from build123d import *

# Parameters (mm, degrees)
RESSALTO_EXTRUS_O1_DEPTH = 37.5


with BuildPart() as part:
    # Esboço1 → Ressalto-extrusão1 (new body, symmetric)
    with BuildSketch(Plane.XY):
        with BuildLine():
            Line((-6, -8.507783687), (-6, -6.707106781))
            Line((-6, -6.707106781), (-4.292893219, -5))
            Line((-4.292893219, -5), (-0.866025404, -5))
            Line((-0.866025404, -5), (0, -4.5))
            Line((0, -4.5), (0.866025404, -5))
            Line((0.866025404, -5), (4.292893219, -5))
            Line((4.292893219, -5), (6, -6.707106781))
            Line((6, -6.707106781), (6, -8.507783687))
            Line((6, -8.507783687), (2.3, -8.507783687))
            Line((2.3, -8.507783687), (2.3, -9.253891844))
            Line((2.3, -9.253891844), (3, -9.253891844))
            Line((3, -9.253891844), (3, -10))
            Line((3, -10), (8.85, -10))
            ThreePointArc((8.85, -10), (9.663172798, -9.663172798), (10, -8.85))
            Line((10, -8.85), (10, -3))
            Line((10, -3), (9.253891844, -3))
            Line((9.253891844, -3), (9.253891844, -2.3))
            Line((9.253891844, -2.3), (8.507783687, -2.3))
            Line((8.507783687, -2.3), (8.507783687, -6))
            Line((8.507783687, -6), (6.707106781, -6))
            Line((6.707106781, -6), (5, -4.292893219))
            Line((5, -4.292893219), (5, -0.867675042))
            Line((5, -0.867675042), (4.502666183, 0))
            Line((4.502666183, 0), (5, 0.866025404))
            Line((5, 0.866025404), (5, 4.292893219))
            Line((5, 4.292893219), (6.707106781, 6))
            Line((6.707106781, 6), (8.507783687, 6))
            Line((8.507783687, 6), (8.507783687, 3))
            Line((8.507783687, 3), (9.253891844, 3))
            Line((9.253891844, 3), (10, 3))
            Line((10, 3), (10, 8.85))
            ThreePointArc((10, 8.85), (9.663172798, 9.663172798), (8.85, 10))
            Line((8.85, 10), (3, 10))
            Line((3, 10), (3, 9.253891844))
            Line((3, 9.253891844), (2.3, 9.253891844))
            Line((2.3, 9.253891844), (2.3, 8.507783687))
            Line((2.3, 8.507783687), (6, 8.507783687))
            Line((6, 8.507783687), (6, 6.707106781))
            Line((6, 6.707106781), (4.292893219, 5))
            Line((4.292893219, 5), (0.866025404, 5))
            Line((0.866025404, 5), (0, 4.502147794))
            Line((0, 4.502147794), (-0.866025404, 5))
            Line((-0.866025404, 5), (-4.292893219, 5))
            Line((-4.292893219, 5), (-6, 6.707106781))
            Line((-6, 6.707106781), (-6, 8.507783687))
            Line((-6, 8.507783687), (-2.3, 8.507783687))
            Line((-2.3, 8.507783687), (-2.3, 9.253891844))
            Line((-2.3, 9.253891844), (-3, 9.253891844))
            Line((-3, 9.253891844), (-3, 10))
            Line((-3, 10), (-8.85, 10))
            ThreePointArc((-8.85, 10), (-9.663172798, 9.663172798), (-10, 8.85))
            Line((-10, 8.85), (-10, 3))
            Line((-10, 3), (-9.253891844, 3))
            Line((-9.253891844, 3), (-9.253891844, 2.3))
            Line((-9.253891844, 2.3), (-8.507783687, 2.3))
            Line((-8.507783687, 2.3), (-8.507783687, 6))
            Line((-8.507783687, 6), (-6.707106781, 6))
            Line((-6.707106781, 6), (-5, 4.292893219))
            Line((-5, 4.292893219), (-5, 0.866025404))
            Line((-5, 0.866025404), (-4.498098017, -0.000824819))
            Line((-4.498098017, -0.000824819), (-5, -0.867675042))
            Line((-5, -0.867675042), (-5, -4.292893219))
            Line((-5, -4.292893219), (-6.707106781, -6))
            Line((-6.707106781, -6), (-8.507783687, -6))
            Line((-8.507783687, -6), (-8.507783687, -2.3))
            Line((-8.507783687, -2.3), (-9.253891844, -2.3))
            Line((-9.253891844, -2.3), (-9.253891844, -3))
            Line((-9.253891844, -3), (-10, -3))
            Line((-10, -3), (-10, -8.85))
            ThreePointArc((-10, -8.85), (-9.663172798, -9.663172798), (-8.85, -10))
            Line((-8.85, -10), (-3, -10))
            Line((-3, -10), (-3, -9.253891844))
            Line((-3, -9.253891844), (-2.3, -9.253891844))
            Line((-2.3, -9.253891844), (-2.3, -8.507783687))
            Line((-2.3, -8.507783687), (-6, -8.507783687))
        make_face()
        with BuildLine():
            Line((-2.445203457, 1.738096676), (-3.181980515, 2.474873734))
            Line((-3.181980515, 2.474873734), (-2.474873734, 3.181980515))
            Line((-2.474873734, 3.181980515), (-1.738096676, 2.445203457))
            ThreePointArc((-1.738096676, 2.445203457), (0, 3), (1.738096676, 2.445203457))
            Line((1.738096676, 2.445203457), (2.474873734, 3.181980515))
            Line((2.474873734, 3.181980515), (3.181980515, 2.474873734))
            Line((3.181980515, 2.474873734), (2.445203457, 1.738096676))
            ThreePointArc((2.445203457, 1.738096676), (3, 0), (2.445203457, -1.738096676))
            Line((2.445203457, -1.738096676), (3.181980515, -2.474873734))
            Line((3.181980515, -2.474873734), (2.474873734, -3.181980515))
            Line((2.474873734, -3.181980515), (1.738096676, -2.445203457))
            ThreePointArc((1.738096676, -2.445203457), (0, -3), (-1.738096676, -2.445203457))
            Line((-1.738096676, -2.445203457), (-2.474873734, -3.181980515))
            Line((-2.474873734, -3.181980515), (-3.181980515, -2.474873734))
            Line((-3.181980515, -2.474873734), (-2.445203457, -1.738096676))
            ThreePointArc((-2.445203457, -1.738096676), (-3, 0), (-2.445203457, 1.738096676))
        make_face(mode=Mode.SUBTRACT)
    extrude(amount=RESSALTO_EXTRUS_O1_DEPTH, both=True)


solid = part.part
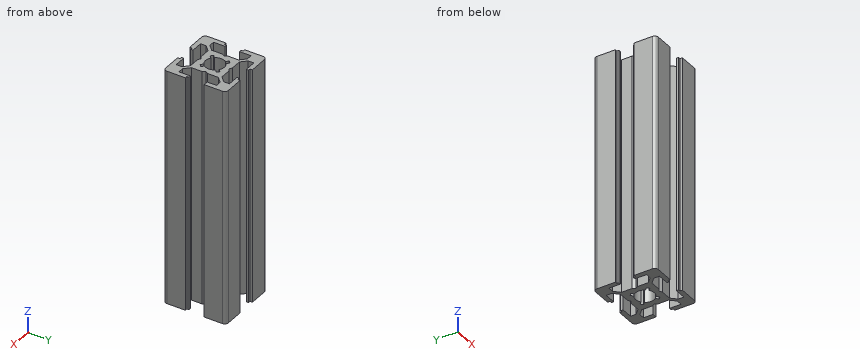
Source: CAD feature listing. Evaluate the final solid. Frame: model axes, mm. Give positions to 0.01 mm unless a question says otherwise; leave off trailing zeros. Write each loop counter-clockwise with the first axis right and the second up, starting at its lowest first coordinate (ties: lowest second). Pieces come first, ordered by that corner, then holes. Notation, with made-up numbers: M 31.5,-34.5 L 79.5,-34.5 A15 cw 79.5,-13.5 Z; hole C -18,45 d1. An arc over 180 degrees is marked long. Return JSON: item names as keys, results as strings. Group by question number.
1) First-contact query: pin 1 Ø0.8 at (x, z) = (-2.5, -5) entering from +Y. Flat tip, straight axial feed; report the tip coordinate or a pass-through.
2) Cut plane A-A, the plane x = 7.75. Output: boundary loops of the cut face in (y, z), then the cut area to 3 significant figures.
3) Ray query, L1, parallel to X at y = -3.5, z = 16; L2, parallel to Y at x = 9, z = -23.5; L3, parallel to Y at x = -7, z = -2.5. Return the intervals inside material, ascending.
Data:
{
 "1": {"pin 1": "stops at y = 9.25"},
 "2": {"outline": "M -10,-37.5 L -6,-37.5 L -6,37.5 L -10,37.5 Z; M 6,-37.5 L 10,-37.5 L 10,37.5 L 6,37.5 Z", "area": "600 mm²"},
 "3": {"L1": "x = -10 to -8.51, -5 to 5, 8.51 to 10", "L2": "y = -9.99 to -2.3, 3 to 9.99", "L3": "y = -10 to -6, 6 to 10"}
}
